Input: dimensioned drawing with shaded views. Units: mm. Origin: part minimum x, y, z. Give positions to 0.01 mm unless a question says otherwise; leave off trailing zeros. Loops run counter-clockwise (first coordinate to the right, second up) from the corner with the lowest first, then second, coordinate; pieces in that order, holes last.
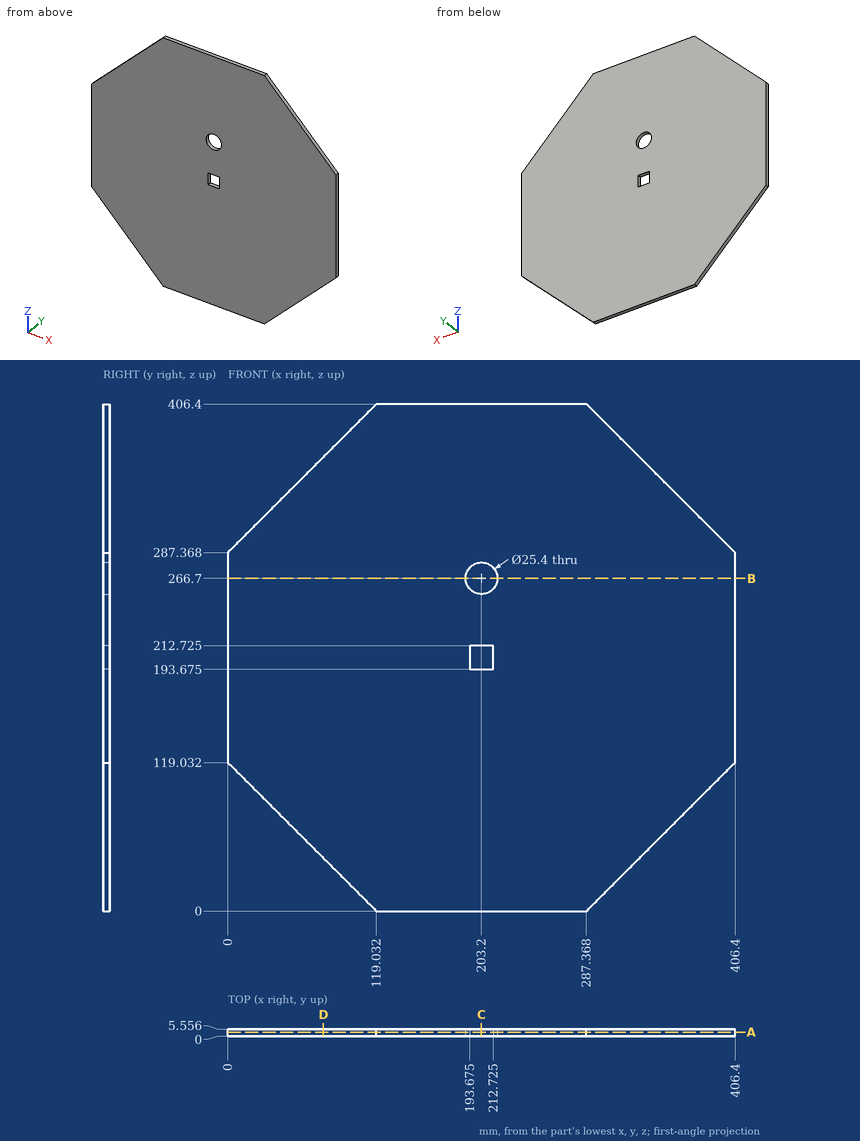
Item 1: Section query D-D on x = 76.5. Return loops of the section in (y, z).
Values follow:
outline: (0, 42.53) - (5.56, 42.53) - (5.56, 363.87) - (0, 363.87) - close
Item 2: Ray query, probe 1 along Z at (x, y) = (203.2, 1.4) (1 decimal); probe 2 along Z at (x, y) = (210, 4) (1 decimal); probe 3 along X at (y, z) = (4.1, 266.7). Return the intervals inside material, ascending.
Values follow:
probe 1: z = 0 to 193.7, 212.7 to 254, 279.4 to 406.4
probe 2: z = 0 to 193.7, 212.7 to 256, 277.4 to 406.4
probe 3: x = 0 to 190.5, 215.9 to 406.4
Item 3: Pin query (flat end, axial travel): pin 1 (2 mm diameter, centred on y = 3.5, z = 290, fed in from +X); pin 2 (1 mm diameter, centred on x = 341, y = 1, fed in from -Z); pin 3 (23 mm diameter, centred on x = 203.2, z = 266.7, fed in from +Y); pin 4 (2 mm diameter, centred on y = 4.5, z = 57, fed in from +X). Return the tip coordinate at first contact, or that it passes through.
Values follow:
pin 1: stops at x = 404.77
pin 2: stops at z = 53.13
pin 3: passes through
pin 4: stops at x = 345.37
Item 4: Section query A-A on y = 3.1. Return loops of the section in (x, z) (1 decimal), plus the area to 3 significant figures.
Values follow:
outline: (0, 119) - (119, 0) - (287.4, 0) - (406.4, 119) - (406.4, 287.4) - (287.4, 406.4) - (119, 406.4) - (0, 287.4) - close; hole circle Ø25.4 at (203.2, 266.7); hole (193.7, 193.7) - (212.7, 193.7) - (212.7, 212.7) - (193.7, 212.7) - close
area: 136,000 mm2
Item 5: Section query B-B on z = 266.7. Return loops of the section in (x, y).
Values follow:
outline: (0, 0) - (190.5, 0) - (190.5, 5.56) - (0, 5.56) - close; (215.9, 0) - (406.4, 0) - (406.4, 5.56) - (215.9, 5.56) - close
Item 6: Section query C-C on x = 203.2. Return loops of the section in (y, z) (1 decimal), plus the area to 3 significant figures.
Values follow:
outline: (0, 0) - (5.6, 0) - (5.6, 193.7) - (0, 193.7) - close; (0, 212.7) - (5.6, 212.7) - (5.6, 254) - (0, 254) - close; (0, 279.4) - (5.6, 279.4) - (5.6, 406.4) - (0, 406.4) - close
area: 2,010 mm2
